Geometry: see drawing. Coordinates: mm, zero at the bounding-box minimum. A direction names the side the tool comes from. Coordinates: 2 decimals unless noted, no trailing zeros. Order: outer loops, then holes, each group sorted by start corner. A loop starts at its lowest first (then second) coordinate and runs counter-clockwise, first axis right, second up.
Item 1: Mould query, pull axis X, two halves, no side actions, for the marked faces 3, 4 and 5. Classes: released by +X, released by -X, zero draft, split by the parting line, or undercut.
Item 2: Contact query for flat-ended pins moving along their axis: P1, Ø10, axis at y = 27, z = 16.5, coming from the -X side; P2, Ø2, axis at x = 13, y = 39.5, coming from the +Z side. Output: stop coordinate, or through.
Item 3: Section B-B on z = 23.25. Return the cut outline in (x, y).
Item 4: Reachability of the marked faces 1 and 2 from +Z, -Z, +X, -X, +Y, -Y: full face, straight path, thin tool, end or side. Return the list, or none.
Item 5: Section A-A on y = 29. Return the cut outline in (x, z).
Item 6: Ray query, line 1 (X direction, y = 29, z = 18); line 2 (Y direction, x = 28, z = 7.5); line 3 (Z direction, x = 5.5, y = 26). Return the intervals inside material, ascending.
Item 7: Section C-C on x = 4.5. Return the cut outline in (y, z).
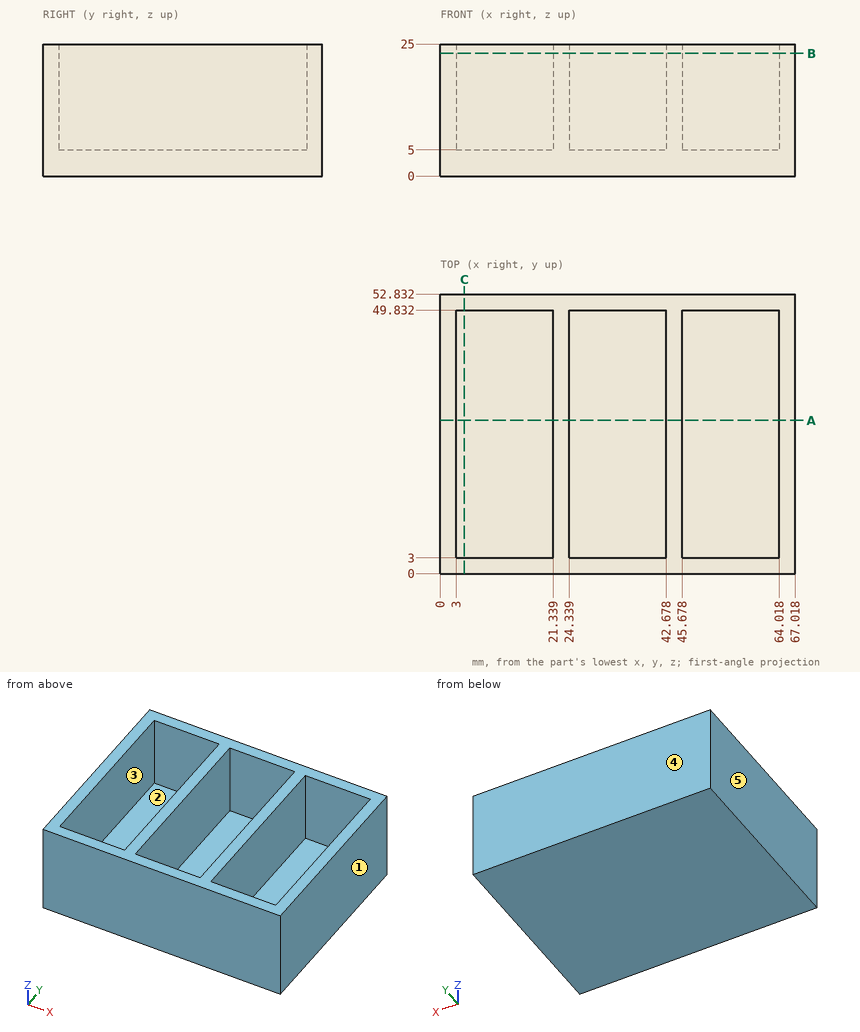
Answer list:
1. face 3: undercut
1. face 4: zero draft
1. face 5: released by -X
2. P1: stops at x = 0
2. P2: stops at z = 5
3. outline: (0, 0) - (67.02, 0) - (67.02, 52.83) - (0, 52.83) - close; hole (3, 3) - (21.34, 3) - (21.34, 49.83) - (3, 49.83) - close; hole (24.34, 3) - (42.68, 3) - (42.68, 49.83) - (24.34, 49.83) - close; hole (45.68, 3) - (64.02, 3) - (64.02, 49.83) - (45.68, 49.83) - close
4. face 1: +Z, -Z, +X, +Y, -Y
4. face 2: +Z
5. outline: (0, 0) - (67.02, 0) - (67.02, 25) - (64.02, 25) - (64.02, 5) - (45.68, 5) - (45.68, 25) - (42.68, 25) - (42.68, 5) - (24.34, 5) - (24.34, 25) - (21.34, 25) - (21.34, 5) - (3, 5) - (3, 25) - (0, 25) - close
6. line 1: x = 0 to 3, 21.34 to 24.34, 42.68 to 45.68, 64.02 to 67.02
6. line 2: y = 0 to 3, 49.83 to 52.83
6. line 3: z = 0 to 5
7. outline: (0, 0) - (52.83, 0) - (52.83, 25) - (49.83, 25) - (49.83, 5) - (3, 5) - (3, 25) - (0, 25) - close
